```python
from build123d import *

# Parameters (mm, degrees)
F0_R        = 1.6
F1_DEPTH    = 2
F2_W        = 2
F2_H        = 50
F3_DEPTH    = 16
F4_R        = 1
F5_T1_DEPTH = 64.1421356237
F6_R        = 3.25
F7_DEPTH    = 25
F8_R        = 5
F10_DEPTH   = 1.5
F12_DEPTH   = 2
F14_DEPTH   = 2


# Not quite as in the source:
# - a fillet or chamfer that OpenCascade refuses, or shapes differently, is made with other operations: its cross-section is extruded or revolved along the edge and cut away or added
# - a feature names something its author has since deleted; it is built from what else it names


with BuildPart() as f1:
    # F0 (on Top) → F1 (new body)
    with BuildSketch(Plane.XY):
        with BuildLine():
            Line((10, 25), (-5, 25))
            ThreePointArc((-5, 25), (-8.5355339059, 23.5355339059), (-10, 20))
            ThreePointArc((-10, 20), (-8.5355339059, 16.4644660941), (-5, 15))
            ThreePointArc((-5, 15), (-1.4644660941, 13.5355339059), (0, 10))
            Line((0, 10), (0, -10))
            ThreePointArc((0, -10), (-1.4644660941, -13.5355339059), (-5, -15))
            ThreePointArc((-5, -15), (-8.5355339059, -16.4644660941), (-10, -20))
            ThreePointArc((-10, -20), (-8.5355339059, -23.5355339059), (-5, -25))
            Line((-5, -25), (10, -25))
            Line((10, -25), (10, 25))
        make_face()
        with Locations((-4, -21)):
            Circle(F0_R, mode=Mode.SUBTRACT)
        with Locations((-4, 21)):
            Circle(F0_R, mode=Mode.SUBTRACT)
    extrude(amount=F1_DEPTH)

    # F2 (on face) → F3 (join)
    with BuildSketch(Plane(origin=(0, 0, 0), x_dir=(1, 0, 0), z_dir=(0, 0, -1))):
        with Locations((4, 0)):
            Rectangle(F2_W, F2_H)
    extrude(amount=F3_DEPTH)

    # F4
    f4_edges = [f1.edges().sort_by_distance(p)[0] for p in [
        (3, 0, 0),
        (5, 0, 0),
    ]]
    fillet(f4_edges, radius=F4_R)

    # F5: fillet of radius 3 on 1 edges, made by hand

    # F5_s2 → F5_t1 (cut)
    with BuildSketch(Plane.XZ.offset(-32.0710678119)):
        with BuildLine():
            ThreePointArc((7.1715728753, 2), (8.9036236828, 1.4494897428), (10, 0))
            Line((10, 0), (10, 2))
            Line((10, 2), (7.1715728753, 2))
        make_face()
    extrude(amount=F5_T1_DEPTH, mode=Mode.SUBTRACT)

    # F6 (on face) → F7 (cut)
    with BuildSketch(Plane.YZ.offset(5)):
        with Locations((-10, -11)):
            Circle(F6_R)
        with Locations((10, -11)):
            Circle(F6_R)
    extrude(amount=-F7_DEPTH, mode=Mode.SUBTRACT)

    # F8
    f8_edges = [f1.edges().sort_by_distance(p)[0] for p in [
        (4, -25, -16),
        (4, 25, -16),
    ]]
    fillet(f8_edges, radius=F8_R)

    # F9 (on Front) → F10 (join, symmetric)
    with BuildSketch(Plane.XZ):
        Polygon((3.4634403419, 0), (0, 0), (3.4634403419, -10.6586683542), align=None)
        Polygon((4.6165082604, -10.6586683542), (9.9565815181, 0), (4.6165082604, 0), align=None)
    extrude(amount=F10_DEPTH, both=True)

    # F11 (on face) → F12 (join)
    with BuildSketch(Plane(origin=(0, 25, 0), x_dir=(-1, 0, 0), z_dir=(0, 1, 0))):
        with BuildLine():
            Line((-3, -5), (0, 0))
            Line((0, 0), (-2, 0))
            ThreePointArc((-2, 0), (-2.7071067812, -0.2928932188), (-3, -1))
            Line((-3, -1), (-3, -5))
        make_face()
        with BuildLine():
            Line((-9.370720014, 0), (-5, -4.2517034346))
            Line((-5, -4.2517034346), (-5, -1))
            ThreePointArc((-5, -1), (-5.2928932188, -0.2928932188), (-6, 0))
            Line((-6, 0), (-9.370720014, 0))
        make_face()
    extrude(amount=-F12_DEPTH)

    # F13 (on face) → F14 (join)
    with BuildSketch(Plane.XZ.offset(25)):
        with BuildLine():
            Line((0, 0), (3, -5))
            Line((3, -5), (3, -1))
            ThreePointArc((3, -1), (2.7071067812, -0.2928932188), (2, 0))
            Line((2, 0), (0, 0))
        make_face()
        with BuildLine():
            Line((5, -1), (5, -4.1425118317))
            Line((5, -4.1425118317), (9.2058293521, 0))
            Line((9.2058293521, 0), (6, 0))
            ThreePointArc((6, 0), (5.2928932188, -0.2928932188), (5, -1))
        make_face()
    extrude(amount=-F14_DEPTH)


solid = f1.part
```
The model under review builds one solid part; all positions refer to its coordinate system, in mm. A direction names the side the tool comes from. Round coordinates to 2 decimals unless told otherwise and drop trailing zeros. Loops run counter-clockwise (first coordinate to the right, second up) from the corner with the lowest first, then second, coordinate; pieces in that order, holes last.
Item 1: Take a section at B-B (x = 3.5). Write out the cut boundary in (y, z).
Determined:
outline: (-25, -11) arc R5 ccw to (-20, -16) - (20, -16) arc R5 ccw to (25, -11) - (25, 2) - (-25, 2) - close; hole circle Ø6.5 at (-10, -11); hole circle Ø6.5 at (10, -11)
Item 2: Clearance check with flat-ended pins moving along their axes: pin 1 Ø3 at (x, z) = (-0.5, -3.5) entering from +Y; pin 2 Ø10 at (x, y) = (-4.5, 6) entering from -Z; pin 3 Ø1.5 at (y, z) = (-17.5, -1) entering from -X; pin 4 Ø0.9 at (x, z) = (1, -4) entering from +Y. State where each tip first meets the part, or that it passes through.
Determined:
pin 1: passes through
pin 2: stops at z = 0
pin 3: stops at x = 2.66
pin 4: stops at y = 1.5
Item 3: For line 1 (Z direction, x = 3.9, y = 10); line 2 (Y direction, x = -4, z = 1); line 3 (X direction, y = -1, z = -13.5), list the stretches that pass through material, from the lowest coordinate up.
Determined:
line 1: z = -16 to -14.25, -7.75 to 2
line 2: y = -25 to -22.6, -19.4 to -14.9, 14.9 to 19.4, 22.6 to 25
line 3: x = 3 to 5
Item 4: For faces 5 (the face through (1.5, 24, -2.5)), 6 (the face through (5, 0.3, -10.1)), 7 (the face through (7.073, -24.014, -2.1)), 8 (the face through (2.699, 12.099, -0.285)), list the 3-axis set-ups (+Z, -Z, +X, -X, +Y, -Y) from which the entire face can be reached by the end or side of a thin tool; tool diameter is ignored.
Determined:
face 5: -Z, -X, +Y
face 6: -Z, +X
face 7: -Z, +X, -Y
face 8: -Z, -X
Item 5: Take a section at A-A (y = 20.5). Write out the cut boundary in (x, z).
Determined:
outline: (-9.97, 0) - (-5.52, 0) - (-5.52, 2) - (-9.97, 2) - close; (-2.48, 0) - (2, 0) arc R1 cw to (3, -1) - (3, -15.97) - (5, -15.97) - (5, -1) arc R1 cw to (6, 0) - (10, 0) arc R3 ccw to (7.17, 2) - (-2.48, 2) - close
Item 6: Take a section at D-D (z = -13.5). Write out the cut boundary in (x, y).
Determined:
outline: (3, -24.33) - (5, -24.33) - (5, -12.08) - (3, -12.08) - close; (3, -7.92) - (5, -7.92) - (5, 7.92) - (3, 7.92) - close; (3, 12.08) - (5, 12.08) - (5, 24.33) - (3, 24.33) - close
Item 7: Mouldability with a two-part tool opening along Z and no side actions: class faces 1 (the face through (3, 0, -10)), 2 (the face through (0.4, 0.4, 2)), 3 (the face through (4.014, -12.395, -8.803)), 4 (the face through (5.301, -12.401, -0.285)) as released by +Z, released by -Z, zero draft, split by the parting line, or undercut.
Determined:
face 1: zero draft
face 2: released by +Z
face 3: undercut
face 4: released by -Z
Item 8: Take a section at C-C (x = -4). Write out the cut boundary in (y, z), then the cut area to 3 significant figures.
Determined:
outline: (-25, 0) - (-22.6, 0) - (-22.6, 2) - (-25, 2) - close; (-19.4, 0) - (-14.9, 0) - (-14.9, 2) - (-19.4, 2) - close; (14.9, 0) - (19.4, 0) - (19.4, 2) - (14.9, 2) - close; (22.6, 0) - (25, 0) - (25, 2) - (22.6, 2) - close
area: 27.6 mm2
